Could you check a few things on this model? Use its own coordinates, in mm. A direction names the side the tool comes from. Round coordinates to 2 decimals unless told otherwise and drop trailing zeros. Write each loop counter-clockwise with the first axis right and the second up, starting at its lowest first coordinate (ties: lowest second). Pieces come first, ordered by that corner, then holes.
```python
from build123d import *

# Parameters (mm, degrees)
EXTRUDE_6_DEPTH     = 10
SKETCH_7_R          = 15
CUT_EXTRUDE_1_DEPTH = 121
SKETCH_8_R          = 4
CUT_EXTRUDE_2_DEPTH = 121


with BuildPart() as part:
    # 草图6 → 凸台-拉伸6 (new body)
    with BuildSketch(Plane.XY.offset(-5)):
        with BuildLine():
            Line((-15, 60), (15, 60))
            Line((15, 60), (15, 20))
            ThreePointArc((15, 20), (16.464466094, 16.464466094), (20, 15))
            Line((20, 15), (60, 15))
            Line((60, 15), (60, -15))
            Line((60, -15), (20, -15))
            ThreePointArc((20, -15), (16.464466094, -16.464466094), (15, -20))
            Line((15, -20), (15, -60))
            Line((15, -60), (-15, -60))
            Line((-15, -60), (-15, -20))
            ThreePointArc((-15, -20), (-16.464466094, -16.464466094), (-20, -15))
            Line((-20, -15), (-60, -15))
            Line((-60, -15), (-60, 15))
            Line((-60, 15), (-20, 15))
            ThreePointArc((-20, 15), (-16.464466094, 16.464466094), (-15, 20))
            Line((-15, 20), (-15, 60))
        make_face()
    extrude(amount=EXTRUDE_6_DEPTH)

    # 草图7 → 切除-拉伸1 (cut, symmetric)
    with BuildSketch(Plane.XY.offset(-5)):
        Circle(SKETCH_7_R)
    extrude(amount=CUT_EXTRUDE_1_DEPTH, both=True, mode=Mode.SUBTRACT)

    # 草图8 → 切除-拉伸2 (cut, symmetric)
    with BuildSketch(Plane.XY.offset(-5)):
        with Locations((45, 0)):
            Circle(SKETCH_8_R)
        with Locations((-45, 0)):
            Circle(SKETCH_8_R)
        with Locations((0, 45)):
            Circle(SKETCH_8_R)
        with Locations((0, -45)):
            Circle(SKETCH_8_R)
    extrude(amount=CUT_EXTRUDE_2_DEPTH, both=True, mode=Mode.SUBTRACT)


solid = part.part
```
Q1. Imagine slicing it at B-B, the plane x = -45. Write out the boundary of the cut face in (y, z), then the cut area to 3 significant figures.
Q2. I'm going to push flat-ended pins straight in: pin 1 Ø5 at (y, z) = (41, 2) entering from -X; pin 2 Ø1.5 at (y, z) = (-36.5, 4) entering from +X; pin 3 Ø3 at (x, z) = (-19, 2) entering from -Y; pin 4 Ø18 at (x, y) = (0, 0) entering from +Z. Where does each tip first touch, or does it pass through?
Q3. On a 3-axis mill with a long thin cutter (end or side, diameter ignored), from which of +Z, -Z, +X, -X, +Y, -Y can I reach the whole of each face in a straight line? I mean faces 4 (the flat face through (40, 15, 0)), 5 (the flat face through (-15, -40, 0)), 6 (the flat face through (40, -15, 0)). Say none if no direction works.
Q4. Imagine slicing it at C-C, the plane z = -0.5. Write out the boundary of the cut face in (x, y), then the cut area to 3 significant figures.
Q5. If I drill on L1, parallel to Y at x = 0, z = -3; L2, parallel to Y at x = 45, z = 2.75; L3, parallel to Y at x = -3.5, z = 2, over which ranges is the centre line in solid material (lowest first)?
Q6. Imagine slicing it at A-A, the plane y = 0. Write out the boundary of the cut face in (x, z), then the cut area to 3 significant figures.
Q7. We'd pull the mould along Y, two halves only. Please class faces 1 (the cylindrical face through (16, 17, 0)), 2 (the flat face through (60, 0, 0)), 3 (the cylindrical face through (1.846, 41.451, -0.07)): pulls with the +Y half, pulls with the -Y half, needs draft (parallel to the pull), parting line crosses it, or undercut.
Results found:
1. outline: (-15, -5) - (-4, -5) - (-4, 5) - (-15, 5) - close; (4, -5) - (15, -5) - (15, 5) - (4, 5) - close
1. area: 220 mm2
2. pin 1: stops at x = -15
2. pin 2: stops at x = 15
2. pin 3: stops at y = -15.67
2. pin 4: passes through
3. face 4: +Z, -Z, +X, +Y
3. face 5: +Z, -Z, -X, -Y
3. face 6: +Z, -Z, +X, -Y
4. outline: (-60, -15) - (-20, -15) arc R5 cw to (-15, -20) - (-15, -60) - (15, -60) - (15, -20) arc R5 cw to (20, -15) - (60, -15) - (60, 15) - (20, 15) arc R5 cw to (15, 20) - (15, 60) - (-15, 60) - (-15, 20) arc R5 cw to (-20, 15) - (-60, 15) - close; hole circle Ø8 at (-45, 0); hole circle Ø30 at (0, 0); hole circle Ø8 at (0, -45); hole circle Ø8 at (0, 45); hole circle Ø8 at (45, 0)
4. area: 5,410 mm2
5. L1: y = -60 to -49, -41 to -15, 15 to 41, 49 to 60
5. L2: y = -15 to -4, 4 to 15
5. L3: y = -60 to -46.94, -43.06 to -14.59, 14.59 to 43.06, 46.94 to 60
6. outline: (-60, -5) - (-49, -5) - (-49, 5) - (-60, 5) - close; (-41, -5) - (-15, -5) - (-15, 5) - (-41, 5) - close; (15, -5) - (41, -5) - (41, 5) - (15, 5) - close; (49, -5) - (60, -5) - (60, 5) - (49, 5) - close
6. area: 740 mm2
7. face 1: pulls with the +Y half
7. face 2: needs draft
7. face 3: undercut
